Can you work these out from the model? Positions are in its coordinate system, mm. Coordinates: 2 decimals unless noted, no trailing zeros. Order: outer loops, then holes, each group sorted by start corner. A loop starts at its lowest first (then second) coordinate and runs counter-clockwise, first axis right, second up. Notation, with made-up numbers: (20.5, 64) -> (69.5, 64) arc R15 cw to (69.5, 68) -> close; hole circle Ø7 at (14.25, 73.25). An arc over 180 degrees is marked (long way). Write item = value, one per line.
```python
from build123d import *

# Parameters (mm, degrees)
SKETCH1_W           = 127.635
SKETCH1_H           = 127.635
BOSS_EXTRUDE1_DEPTH = 12.7
SKETCH12_R          = 95.4151
BOSS_EXTRUDE2_DEPTH = 12.7
SKETCH5_R           = 46.355
CUT_EXTRUDE1_DEPTH  = 9.525
SKETCH30_R          = 85.09
SKETCH30_R_2        = 79.375
BOSS_EXTRUDE3_DEPTH = 12.7
SKETCH32_R          = 1.35255
CUT_EXTRUDE4_DEPTH  = 15.24
CIRPATTERN2_COUNT   = 12
SKETCH36_R          = 115.31206939
SKETCH36_R_2        = 76.2
CUT_EXTRUDE5_DEPTH  = 35.9250001
SKETCH38_R          = 95.25
SKETCH38_R_2        = 76.2
BOSS_EXTRUDE4_DEPTH = 12.7
SKETCH37_W          = 208.61583397
SKETCH37_H          = 123.882270127
CUT_EXTRUDE6_DEPTH  = 96.25


with BuildPart() as part:
    # Sketch1 → Boss-Extrude1 (new body)
    with BuildSketch(Plane(origin=(0, 0, 0), x_dir=(1, 0, 0), z_dir=(0, 1, 0))):
        with Locations((63.8175, 63.8175)):
            Rectangle(SKETCH1_W, SKETCH1_H)
    extrude(amount=BOSS_EXTRUDE1_DEPTH)

    # Sketch12 → Boss-Extrude2 (add)
    with BuildSketch(Plane.XZ):
        with Locations((63.8175, -63.8175)):
            Circle(SKETCH12_R)
    extrude(amount=-BOSS_EXTRUDE2_DEPTH)

    # Sketch5 → Cut-Extrude1 (cut)
    with BuildSketch(Plane(origin=(0, 12.7, 0), x_dir=(1, 0, 0), z_dir=(0, 1, 0))):
        with Locations((63.8175, 63.8175)):
            Circle(SKETCH5_R)
    extrude(amount=-CUT_EXTRUDE1_DEPTH, mode=Mode.SUBTRACT)

    # Sketch30 → Boss-Extrude3 (add)
    with BuildSketch(Plane.XZ):
        with Locations((63.8175, -63.8175)):
            Circle(SKETCH30_R)
        with Locations((63.8175, -63.8175)):
            Circle(SKETCH30_R_2, mode=Mode.SUBTRACT)
    boss_extrude3 = extrude(amount=BOSS_EXTRUDE3_DEPTH)

    # Mirror1: Boss-Extrude3 across plane
    add(boss_extrude3.mirror(Plane.ZX.offset(4.7625)))

    # Sketch32 → Cut-Extrude4 (cut)
    with BuildSketch(Plane(origin=(0, 0, -148.9075), x_dir=(-1, 0, 0), z_dir=(0, 0, -1))):
        with Locations((-63.8175, -6.35)):
            Circle(SKETCH32_R)
        with Locations((-63.8175, 19.05)):
            Circle(SKETCH32_R)
    cut_extrude4 = extrude(amount=-CUT_EXTRUDE4_DEPTH, mode=Mode.SUBTRACT)

    # CirPattern2: Cut-Extrude4 ×12 about axis
    cirpattern2_axis = Axis((63.8175, -12.7, -63.8175), (0, 1, 0))
    for i in range(1, CIRPATTERN2_COUNT):
        add(cut_extrude4.rotate(cirpattern2_axis, i * 360 / CIRPATTERN2_COUNT), mode=Mode.SUBTRACT)

    # Sketch35 → Cut-Revolve1 (revolve, cut)
    with BuildSketch(Plane.XY.offset(-63.754)):
        with BuildLine():
            add(Edge.make_bspline(
                [(129.8575, 12.7), (125.556720128, 5.300210603), (116.945262531, 3.999403305), (110.1725, 0)],
                knots=[0, 0, 0, 0, 1, 1, 1, 1], degree=3))
            Line((110.1725, 0), (63.8175, 0))
            Line((63.8175, 0), (63.8175, 12.7))
            Line((63.8175, 12.7), (129.8575, 12.7))
        make_face()
    revolve(axis=Axis((63.8175, -10.330163638, -63.754), (0, 1, 0)), mode=Mode.SUBTRACT)

    # Sketch36 → Cut-Extrude5 (cut, through all)
    with BuildSketch(Plane(origin=(0, 22.225, 0), x_dir=(1, 0, 0), z_dir=(0, 1, 0))):
        with Locations((63.8175, 63.8175)):
            Circle(SKETCH36_R)
        with Locations((63.8175, 63.8175)):
            Circle(SKETCH36_R_2, mode=Mode.SUBTRACT)
    extrude(amount=-CUT_EXTRUDE5_DEPTH, mode=Mode.SUBTRACT)

    # Sketch38 → Boss-Extrude4 (add)
    with BuildSketch(Plane(origin=(0, 0, 0), x_dir=(-1, 0, 0), z_dir=(0, -1, 0))):
        with Locations((-63.8175, 63.8175)):
            Circle(SKETCH38_R)
        with Locations((-63.8175, 63.8175)):
            Circle(SKETCH38_R_2, mode=Mode.SUBTRACT)
    extrude(amount=-BOSS_EXTRUDE4_DEPTH)

    # Sketch37 → Cut-Extrude6 (cut, through all)
    with BuildSketch(Plane(origin=(63.8175, 0, 0), x_dir=(0, 0, -1), z_dir=(-1, 0, 0))):
        with Locations((61.023743595, -14.657491218)):
            Rectangle(SKETCH37_W, SKETCH37_H)
    extrude(amount=-CUT_EXTRUDE6_DEPTH, mode=Mode.SUBTRACT)


solid = part.part
```
Item 1: If I drill on probe 1 along Z at (x, y) = (12.5, 10.75); probe 2 along Z at (x, y) = (23, 11.5); probe 3 along X at (y, z) = (6.75, -129.5), over which ranges is the centre line in solid material (lowest first)?
A:
probe_1 = -144.06 to -103.16, -24.34 to 16.43
probe_2 = -149.88 to -114.69, -12.82 to 22.24
probe_3 = -5.16 to 63.82
Item 2: I'm going to push flat-ended pins straight in: P1, Ø1.5, axis at x = 21, z = -40, coming from the +Y side; P2, Ø3, axis at y = 6, z = -41, coming from the -X side; P3, Ø2, axis at x = 19.5, z = -44.5, coming from the +Y side. Where does each tip first touch, or does it pass through?
A:
P1 = 1.75
P2 = -29.02
P3 = 1.56
Item 3: I want a section at A-A, the plane x = -4.5. Please give me the cut outline in (y, z).
A:
outline = (0, -130.19) -> (12.7, -130.19) -> (12.7, 2.55) -> (0, 2.55) -> close
Item 4: I want a section at B-B, the plane z = 15. Please give me the cut outline in (x, y), plus the area to 3 significant figures.
A:
outline = (10.34, 0) -> (63.82, 0) -> (63.82, 12.7) -> (10.34, 12.7) -> close
area = 679 mm2
